```python
from build123d import *

# Parameters (mm, degrees)
SKETCH_1_W          = 10.5
SKETCH_1_H          = 38.1
EXTRUDE_1_DEPTH     = 30
SKETCH_2_R          = 2
CUT_EXTRUDE_1_DEPTH = 11
SKETCH_3_R          = 1.8
CUT_EXTRUDE_2_DEPTH = 17
SKETCH_4_R          = 1.8
CUT_EXTRUDE_3_DEPTH = 9
SKETCH_5_W          = 10.5
SKETCH_5_H          = 7.5
CUT_EXTRUDE_4_DEPTH = 30


with BuildPart() as part:
    # 草圖1 → 填料-伸長1 (new body)
    with BuildSketch(Plane(origin=(0, 0, 0), x_dir=(1, 0, 0), z_dir=(0, 1, 0))):
        with Locations((5.25, 19.05)):
            Rectangle(SKETCH_1_W, SKETCH_1_H)
    extrude(amount=EXTRUDE_1_DEPTH)

    # 草圖2 → 除料-伸長1 (cut)
    with BuildSketch(Plane(origin=(10.5, 0, 0), x_dir=(0, 0, -1), z_dir=(1, 0, 0))):
        with Locations((22, 24)):
            Circle(SKETCH_2_R)
        with Locations((22, 16)):
            Circle(SKETCH_2_R)
        with Locations((22, 8)):
            Circle(SKETCH_2_R)
    extrude(amount=-CUT_EXTRUDE_1_DEPTH, mode=Mode.SUBTRACT)

    # 草圖3 → 除料-伸長2 (cut)
    with BuildSketch(Plane.XY):
        with Locations((5.25, 23)):
            Circle(SKETCH_3_R)
        with Locations((5.25, 15)):
            Circle(SKETCH_3_R)
        with Locations((5.25, 7)):
            Circle(SKETCH_3_R)
    extrude(amount=-CUT_EXTRUDE_2_DEPTH, mode=Mode.SUBTRACT)

    # 草圖4 → 除料-伸長3 (cut)
    with BuildSketch(Plane(origin=(0, 0, -38.1), x_dir=(-1, 0, 0), z_dir=(0, 0, -1))):
        with Locations((-6.25, 26)):
            Circle(SKETCH_4_R)
        with Locations((-6.25, 18)):
            Circle(SKETCH_4_R)
        with Locations((-6.25, 10)):
            Circle(SKETCH_4_R)
    extrude(amount=-CUT_EXTRUDE_3_DEPTH, mode=Mode.SUBTRACT)

    # 草圖5 → 除料-伸長4 (cut)
    with BuildSketch(Plane(origin=(0, 30, 0), x_dir=(1, 0, 0), z_dir=(0, 1, 0))):
        with Locations((5.25, 3.75)):
            Rectangle(SKETCH_5_W, SKETCH_5_H)
    extrude(amount=-CUT_EXTRUDE_4_DEPTH, mode=Mode.SUBTRACT)


solid = part.part
```
Part model, mm, in its own coordinate system. A direction names the side the tool comes from. Round coordinates to 2 decimals unless told otherwise and drop trailing zeros. Loops run counter-clockwise (first coordinate to the right, second up) from the corner with the lowest first, then second, coordinate; pieces in that order, holes last.
Item 1: Cut at C-C, the plane z = -21.5. Give the cut face in (x, y), then the cut area to 3 significant figures.
Item 2: Mould opens along Z. For faces 4 (the face through (5, 7, -17)), 5 (the face through (5, 30, -23)), 6 (the face through (5.3, 22.8, -20.4)), 7 (the face through (5, 15, -38.1)) say: +Z half, -Z half, draft (parallel to the pull), parting line (faces both ways), or undercut.
Item 3: Drill centre lines: line 1 (Y direction, x = 5.25, z = -14); line 2 (Y direction, x = 6.25, z = -33); line 3 (Z direction, x = 7.5, y = 17.5). Where is each one in solid material? Low to high.
Item 4: Cut at D-D, the plane y = 15. Give the cut face in (x, z).
Item 5: Cut at A-A, the plane z = -32. Give the cut face in (x, y).
Item 6: Drop flat-ended pins along their axis: P1, Ø1.8, axis at x = 6, y = 10.5, coming from the -Z side; P2, Ø3, axis at x = 5.25, y = 7, coming from the +Z side. Give the stop position or say it passes through.
Item 7: 3-axis set-ups, long thin cutter, end or side, ignore diameter. For faces 1 (the face through (3, 15, -7.5)), 2 (the face through (6.218, 24.518, -12.183)), 3 (the face through (6, 26, -29.1)): which of +Z, -Z, +X, -X, +Y, -Y reach the whole face in a straight line?
Item 8: Cut at B-B, the plane x = 1. Give the cut face in (y, z).
A:
1. outline: (0, 0) - (10.5, 0) - (10.5, 6.06) - (0, 6.06) - close; (0, 9.94) - (10.5, 9.94) - (10.5, 14.06) - (0, 14.06) - close; (0, 17.94) - (10.5, 17.94) - (10.5, 22.06) - (0, 22.06) - close; (0, 25.94) - (10.5, 25.94) - (10.5, 30) - (0, 30) - close
1. area: 193 mm2
2. face 4: +Z half
2. face 5: draft
2. face 6: undercut
2. face 7: -Z half
3. line 1: y = 0 to 5.2, 8.8 to 13.2, 16.8 to 21.2, 24.8 to 30
3. line 2: y = 0 to 8.2, 11.8 to 16.2, 19.8 to 24.2, 27.8 to 30
3. line 3: z = -29.1 to -23.32, -20.68 to -7.5
4. outline: (0, -38.1) - (10.5, -38.1) - (10.5, -23.73) - (0, -23.73) - close; (0, -20.27) - (10.5, -20.27) - (10.5, -7.5) - (7.05, -7.5) - (7.05, -17) - (3.45, -17) - (3.45, -7.5) - (0, -7.5) - close
5. outline: (0, 0) - (10.5, 0) - (10.5, 30) - (0, 30) - close; hole circle Ø3.6 at (6.25, 10); hole circle Ø3.6 at (6.25, 18); hole circle Ø3.6 at (6.25, 26)
6. P1: stops at z = -29.1
6. P2: stops at z = -17
7. face 1: +Z, +X, -X, +Y, -Y
7. face 2: +Z
7. face 3: -Z
8. outline: (0, -38.1) - (30, -38.1) - (30, -7.5) - (0, -7.5) - close; hole circle Ø4 at (8, -22); hole circle Ø4 at (16, -22); hole circle Ø4 at (24, -22)
